Can you work these out from the model? Positions are in its coordinate system, mm. Face numbers are marked on the shaded views. A direction names the side the tool comes from. Give positions to 0.01 mm unless a question says otherwise; leave off trailing zeros. Order: outer loops, then holes, each group sorted by start corner. A loop starts at its lowest first (then second) coordinate and runs counter-clockwise, first axis right, second up.
Item 1: I want a section at B-B, the plane z = 86. Write out the boundary of the cut face in (x, y), then the cut area to 3 significant figures.
Item 2: I'm going to push flat-ended pins straight in: pin 1 Ø4 at (y, z) = (-64, -4.5) entering from -X; pin 2 Ø11.5 at (y, z) = (-117, 45) entering from +X; pin 3 Ø22 at (x, y) = (71.5, -79) entering from +Z. Where does each tip first touch, or does it pass through?
Item 3: If I drill on line 1 along Y through (x, z) = (32.5, 31); line 2 along X through (y, z) = (-109, 23); line 3 along Z through (x, y) = (15.5, -32), over which ranges is the centre line in solid material (lowest first)?
Item 4: Which directions (+Z, -Z, +X, -X, +Y, -Y) give clear straight access to the entire face, cutting with the end or side of a thin tool? Please do the marked faces 5, 6 and 7.
Item 5: I want a section at A-A, the plane x = -0.5. Write out the boundary of the cut face in (y, z), then the cut area to 3 significant figures.
Item 6: If we mould it in two halves opening along Y, with no side actions, what happens to the marked faces 1, 2, 3 and 4? For each: +Y half, -Y half, draft (parallel to the pull), parting line (faces both ways), or undercut.
Item 7: I want a section at D-D, the plane x = 80. Write out the boundary of the cut face in (y, z), then the cut area to 3 significant figures.
Item 8: I want a section at C-C, the plane y = -62.5. Write out the boundary of the cut face in (x, z).
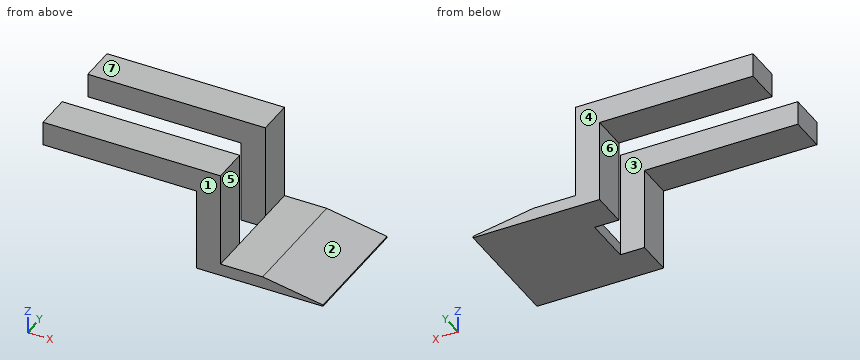
```python
from build123d import *

# Parameters (mm, degrees)
F1_DEPTH = 127
F2_W     = 186.9721719681
F2_H     = 50.8
F3_DEPTH = 112.5370903122
F4_SIZE2 = 11.196763275
F4_SIZE  = 63.5


with BuildPart() as f1:
    # F0 (on Front) → F1 (new body)
    with BuildSketch(Plane.XZ):
        Polygon((162.2777349776, -12.7), (162.2777349776, 0), (54.3277631103, 0), (54.3277631103, 99.8360903122), (-132.6444088578, 99.8360903122), (-132.6444088578, 74.4360903122), (28.9277631103, 74.4360903122), (28.9277631103, -12.7), align=None)
    extrude(amount=F1_DEPTH)

    # F2 (on face) → F3 (cut, through all)
    with BuildSketch(Plane.XY.offset(99.8360903122)):
        with Locations((-39.1583228738, -63.5)):
            Rectangle(F2_W, F2_H)
    extrude(amount=-F3_DEPTH, mode=Mode.SUBTRACT)

    # F4
    f4_edges = [f1.edges().sort_by_distance(p)[0] for p in [
        (162.277735, -63.5, 0),
    ]]
    f4_side = f1.faces().sort_by_distance((108.302749, -63.5, 0))[0]
    chamfer(f4_edges, length=F4_SIZE, length2=F4_SIZE2, reference=f4_side)


solid = f1.part
```
Results list:
1. outline: (-132.64, -127) - (54.33, -127) - (54.33, -88.9) - (-132.64, -88.9) - close; (-132.64, -38.1) - (54.33, -38.1) - (54.33, 0) - (-132.64, 0) - close
1. area: 14,200 mm2
2. pin 1: stops at x = 54.33
2. pin 2: stops at x = 54.33
2. pin 3: stops at z = 0
3. line 1: y = -127 to -88.9, -38.1 to 0
3. line 2: x = 28.93 to 54.33
3. line 3: z = 74.44 to 99.84
4. face 5: +Z, +X, +Y, -Y
4. face 6: -Z, -X, +Y, -Y
4. face 7: +Z, +X, -X, +Y, -Y
5. outline: (-127, 74.44) - (-88.9, 74.44) - (-88.9, 99.84) - (-127, 99.84) - close; (-38.1, 74.44) - (0, 74.44) - (0, 99.84) - (-38.1, 99.84) - close
5. area: 1,940 mm2
6. face 1: -Y half
6. face 2: draft
6. face 3: undercut
6. face 4: +Y half
7. outline: (-127, -12.7) - (0, -12.7) - (0, 0) - (-127, 0) - close
7. area: 1,610 mm2
8. outline: (54.33, -12.7) - (162.28, -12.7) - (162.28, -11.2) - (98.78, 0) - (54.33, 0) - close
